Model file for the job. Use its own axes, mm. A direction names the side the tool comes from. Give positions to 0.01 mm unless a question says otherwise; leave off trailing zeros. Write each loop counter-clockwise with the first axis right and the second up, starting at its lowest first coordinate (ties: lowest second). Pieces come first, ordered by that corner, then holes.
```python
from build123d import *

# Parameters (mm, degrees)
SKETCH1_W                  = 298.45
SKETCH1_H                  = 495.3
BOSS_EXTRUDE1_DEPTH        = 4.7625
CUT_EXTRUDE1_DEPTH         = 290.291114191
CUT_EXTRUDE1_DEPTH_BACK    = 290.291114191
SKETCH3_W                  = 196.85
SKETCH3_H                  = 114.3
SKETCH20_W                 = 47.879
SKETCH20_H                 = 47.879
CUT_EXTRUDE5_DEPTH         = 290.291114191
F_10_CLEARANCE_HOLE1_D     = 5.1054
F_10_CLEARANCE_HOLE1_DEPTH = 10.668
F_10_CLEARANCE_HOLE1_TIP   = 1.533816902
F_10_CLEARANCE_HOLE4_D     = 5.1054
LPATTERN3_COUNT            = 3
LPATTERN3_PITCH            = 63.5
MIRROR2_COPY_1_D           = 5.1054
MIRROR2_COPY_2_D           = 5.1054
F_10_CLEARANCE_HOLE5_D     = 5.1054
LPATTERN4_COUNT            = 3
LPATTERN4_PITCH            = 96.52
LPATTERN4_COL_COUNT        = 3
LPATTERN4_COL_PITCH        = 96.52
MIRROR3_COPY_1_D           = 5.1054
MIRROR3_COPY_2_D           = 5.1054
MIRROR3_COPY_3_D           = 5.1054
MIRROR3_COPY_4_D           = 5.1054
F_10_CLEARANCE_HOLE6_D     = 5.1054
F_10_CLEARANCE_HOLE7_D     = 5.1054


with BuildPart() as part:
    # Sketch1 → Boss-Extrude1 (new, symmetric)
    with BuildSketch(Plane(origin=(0, 0, 0), x_dir=(1, 0, 0), z_dir=(0, 1, 0))):
        Rectangle(SKETCH1_W, SKETCH1_H)
    extrude(amount=BOSS_EXTRUDE1_DEPTH, both=True)

    # Sketch3 → Cut-Extrude1 (cut, two sides: drawn at the far end of the back side and taken through both)
    with BuildSketch(Plane(origin=(0, 4.7625, 0), x_dir=(1, 0, 0), z_dir=(0, 1, 0)).offset(-CUT_EXTRUDE1_DEPTH_BACK)):
        with Locations((0, -44.45)):
            Rectangle(SKETCH3_W, SKETCH3_H)
    extrude(amount=CUT_EXTRUDE1_DEPTH + CUT_EXTRUDE1_DEPTH_BACK, mode=Mode.SUBTRACT)

    # Sketch20 → Cut-Extrude5 (cut, through all)
    with BuildSketch(Plane.XZ.offset(4.7625)):
        with Locations((0, 171.45)):
            Rectangle(SKETCH20_W, SKETCH20_H)
    extrude(amount=-CUT_EXTRUDE5_DEPTH, mode=Mode.SUBTRACT)

    # #10 Clearance Hole1
    with Locations(Plane(origin=(0, -4.7625, 0), x_dir=(-1, 0, 0), z_dir=(0, -1, 0))):
        with Locations((-38.1, -155.575), (38.1, -155.575), (38.1, -187.325), (-38.1, -187.325)):
            Hole(F_10_CLEARANCE_HOLE1_D / 2, depth=F_10_CLEARANCE_HOLE1_DEPTH)
            with Locations((0, 0, -(F_10_CLEARANCE_HOLE1_DEPTH + F_10_CLEARANCE_HOLE1_TIP / 2))):  # 118° drill point
                Cone(0, F_10_CLEARANCE_HOLE1_D / 2, F_10_CLEARANCE_HOLE1_TIP, mode=Mode.SUBTRACT)

    # #10 Clearance Hole4 (through all)
    with Locations(Plane(origin=(0, 4.7625, 0), x_dir=(1, 0, 0), z_dir=(0, 1, 0))):
        with Locations((-63.5, 241.3)):
            f_10_clearance_hole4 = Hole(F_10_CLEARANCE_HOLE4_D / 2)

    # LPattern3: #10 Clearance Hole4 ×3
    with Locations(*[(i * LPATTERN3_PITCH, 0, 0) for i in range(1, LPATTERN3_COUNT)]):
        add(f_10_clearance_hole4, mode=Mode.SUBTRACT)

    # Mirror2: #10 Clearance Hole4 across plane
    add(f_10_clearance_hole4.mirror(Plane.XY), mode=Mode.SUBTRACT)

    # Mirror2 copy 1 (through all)
    with Locations(Plane(origin=(63.5, 4.7625, 0), x_dir=(1, 0, 0), z_dir=(0, 1, 0))):
        with Locations((-63.5, -241.3)):
            Hole(MIRROR2_COPY_1_D / 2)

    # Mirror2 copy 2 (through all)
    with Locations(Plane(origin=(127, 4.7625, 0), x_dir=(1, 0, 0), z_dir=(0, 1, 0))):
        with Locations((-63.5, -241.3)):
            Hole(MIRROR2_COPY_2_D / 2)

    # #10 Clearance Hole5 (through all)
    with Locations(Plane(origin=(0, 4.7625, 0), x_dir=(1, 0, 0), z_dir=(0, 1, 0))):
        with Locations((-142.875, 0)):
            f_10_clearance_hole5 = Hole(F_10_CLEARANCE_HOLE5_D / 2)

    # LPattern4: #10 Clearance Hole5 ×3
    with Locations(*[(0, 0, -i * LPATTERN4_PITCH) for i in range(1, LPATTERN4_COUNT)]):
        add(f_10_clearance_hole5, mode=Mode.SUBTRACT)

    # LPattern4 col: #10 Clearance Hole5 ×3
    with Locations(*[(0, 0, i * LPATTERN4_COL_PITCH) for i in range(1, LPATTERN4_COL_COUNT)]):
        add(f_10_clearance_hole5, mode=Mode.SUBTRACT)

    # Mirror3: #10 Clearance Hole5 across plane
    add(f_10_clearance_hole5.mirror(Plane(origin=(0, 0, 0), x_dir=(0, 0, 1), z_dir=(1, 0, 0))), mode=Mode.SUBTRACT)

    # Mirror3 copy 1 (through all)
    with Locations(Plane(origin=(0, 4.7625, -96.52), x_dir=(-1, 0, 0), z_dir=(0, 1, 0))):
        with Locations((-142.875, 0)):
            Hole(MIRROR3_COPY_1_D / 2)

    # Mirror3 copy 2 (through all)
    with Locations(Plane(origin=(0, 4.7625, -193.04), x_dir=(-1, 0, 0), z_dir=(0, 1, 0))):
        with Locations((-142.875, 0)):
            Hole(MIRROR3_COPY_2_D / 2)

    # Mirror3 copy 3 (through all)
    with Locations(Plane(origin=(0, 4.7625, 96.52), x_dir=(-1, 0, 0), z_dir=(0, 1, 0))):
        with Locations((-142.875, 0)):
            Hole(MIRROR3_COPY_3_D / 2)

    # Mirror3 copy 4 (through all)
    with Locations(Plane(origin=(0, 4.7625, 193.04), x_dir=(-1, 0, 0), z_dir=(0, 1, 0))):
        with Locations((-142.875, 0)):
            Hole(MIRROR3_COPY_4_D / 2)

    # #10 Clearance Hole6 (through all)
    with Locations(Plane(origin=(0, 4.7625, 0), x_dir=(1, 0, 0), z_dir=(0, 1, 0))):
        with Locations((120.65, 39.4255), (120.65, -114.6255), (-120.65, -114.6255), (-120.65, 39.4255)):
            Hole(F_10_CLEARANCE_HOLE6_D / 2)

    # #10 Clearance Hole7 (through all)
    with Locations(Plane(origin=(0, 4.7625, 0), x_dir=(1, 0, 0), z_dir=(0, 1, 0))):
        with Locations((76.2, 33.0755), (0, 33.0755), (-76.2, 33.0755), (-76.2, -120.9755), (0, -120.9755), (76.2, -120.9755)):
            Hole(F_10_CLEARANCE_HOLE7_D / 2)


solid = part.part
```
1. Slice it at B-B, the plane x = -92.5. Write the cut outline in (y, z), and give its area (3 significant figures).
Calculated:
outline: (-4.76, -247.65) - (4.76, -247.65) - (4.76, -12.7) - (-4.76, -12.7) - close; (-4.76, 101.6) - (4.76, 101.6) - (4.76, 247.65) - (-4.76, 247.65) - close
area: 3,630 mm2
2. Which spindle directions (+Z, -Z, +X, -X, +Y, -Y) get a long thin tool onto all of the face, cutting with end or side? Do faces 1 (the flat face through (-23.94, 0, 171)), 2 (the flat face through (-2, 4.762, -59)). Say none if no direction does.
Calculated:
face 1: +Y, -Y
face 2: +Z, -Z, +X, -X, +Y
3. Slice it at C-C, the plane y = -0.5. State how many separate pieces and enclosed holes the cut face has, and give its area (3 significant figures).
Calculated:
separate pieces: 1
enclosed holes: 32
area: 122,000 mm2
4. Probe probe 1 along Z at (x, y) = (-76.2, 3.25); probe 2 along X at (y, z) = (4.25, 62) (3 decimals); probe 3 along Z at (x, y) = (-38.1, -1). List the from-to ranges inside material, lowest first.
Calculated:
probe 1: z = -247.65 to -35.63, -30.52 to -12.7, 101.6 to 118.42, 123.53 to 247.65
probe 2: x = -149.225 to -98.425, 98.425 to 149.225
probe 3: z = -247.65 to -12.7, 101.6 to 153.02, 158.13 to 184.77, 189.88 to 247.65
5. Pull direction X, two halves, no side cores. Call faces 3 (the flat face through (-2, 0, 247.65)), 4 (the flat face through (23.94, 0, 171)), 5 (the flat face through (-149.225, 0, 3)): +X half, -X half, draft (parallel to the pull), parting line (faces both ways), or undercut.
Calculated:
face 3: draft
face 4: undercut
face 5: -X half
6. Slice it at A-A, the plane z = 74.5. Write the cut outline in (x, y) (1 decimal).
Calculated:
outline: (-149.2, -4.8) - (-98.4, -4.8) - (-98.4, 4.8) - (-149.2, 4.8) - close; (98.4, -4.8) - (149.2, -4.8) - (149.2, 4.8) - (98.4, 4.8) - close
